```python
from build123d import *

# Parameters (mm, degrees)
GOBLET_SHELL_T                     = -4
SKETCH2_R                          = 44
CUT_TO_FIT_WITH_BLADE_CASING_DEPTH = 10


with BuildPart() as part:
    # Sketch1 → Goblet Revolve (revolve)
    with BuildSketch(Plane.XY, mode=Mode.PRIVATE) as goblet_revolve_sk:
        Polygon((0, 0), (48, 0), (48, 8), (60, 8), (60, 136), (0, 136), align=None)
    revolve(goblet_revolve_sk.sketch.rotate(Axis((0, 136, 0), (0, -1, 0)), 90), axis=Axis((0, 136, 0), (0, -1, 0)))

    # Goblet Shell
    goblet_shell_openings = [part.faces().sort_by_distance(p)[0] for p in [
        (0, 136, 0),
    ]]
    offset(amount=GOBLET_SHELL_T, openings=goblet_shell_openings, kind=Kind.INTERSECTION)

    # Sketch2 → Cut to Fit with Blade Casing (cut)
    with BuildSketch(Plane(origin=(0, 4, 0), x_dir=(1, 0, 0), z_dir=(0, 1, 0))):
        with Locations(Location((0, 0, 0), (0, 0, 270))):
            Circle(SKETCH2_R)
    extrude(amount=-CUT_TO_FIT_WITH_BLADE_CASING_DEPTH, mode=Mode.SUBTRACT)


solid = part.part
```
Geometry: final body of the model. Coordinates: model frame, mm. A direction names the side the tool comes from. Round coordinates to 2 decimals unless told otherwise and drop trailing zeros. Order: outer loops, then holes, each group sorted by start corner. A loop starts at its lowest first (then second) coordinate and runs counter-clockwise, first axis right, second up. Notation, with made-up numbers: (0.5, 80) -> (58.5, 80) arc R31 cw to (58.5, 116) -> close; hole circle Ø2 at (-39.5, -22). An arc over 180 degrees is marked (long way). Use one line per item in the form item = value. Start each with the question number.
1. Cut plane B-B (z = 0). Return the cut outline in (x, y), then the cut area to 3 significant figures.
2. Cut plane C-C (y = 50.5). Return the cut outline in (x, z), then the cut area to 3 significant figures.
3. Cut plane A-A (x = 0). Return the cut outline in (y, z).
4. Draft query along X for faces 1 (the face through (49.68, 74.87, 25.84)), 2 (the face through (-50.59, 72.9, 32.26)), 3 (the face through (-40, 8, 27)). Return one class per face: pulls with the +X half, pulls with the -X half, needs draft (parallel to the pull), parting line crosses it, or undercut.
5. Line query: probe 1 along X at (y, z) = (1.3, 0); probe 2 along Z at (x, y) = (-2, 114.5); probe 3 along X at (y, z) = (86, 0). Output: solid intervals per line, ascending.
6. Cut plane D-D (x = 52). Return the cut outline in (y, z).
7. Reachability of faces 4 (the face through (37, 12, -25)), 5 (the face through (-14.418, 4.056, 45.783)), 6 (the face through (40, 136, 40)) from +Z, -Z, +X, -X, +Y, -Y: full face, straight path, thin tool, end or side. Return the list, or none.
8. Pin query (flat end, axial travel): pin 1 Ø10 at (x, z) = (45.5, 2) entering from +Y; pin 2 Ø5 at (y, z) = (107, -11) entering from -X; pin 3 Ø8 at (x, z) = (7.5, -39) entering from -Y; pin 4 Ø8 at (x, y) = (26.5, 18.5) entering from +Z. Return the tip coordinate at first contact, or that it passes through.
Solution:
q1.outline = (-60, 8) -> (-48, 8) -> (-48, 0) -> (-44, 0) -> (-44, 12) -> (-56, 12) -> (-56, 136) -> (-60, 136) -> close; (44, 0) -> (48, 0) -> (48, 8) -> (60, 8) -> (60, 136) -> (56, 136) -> (56, 12) -> (44, 12) -> close
q1.area = 1,180 mm^2
q2.outline = circle Ø120 at (0, 0); hole circle Ø112 at (0, 0)
q2.area = 1,460 mm^2
q3.outline = (0, -48) -> (8, -48) -> (8, -60) -> (136, -60) -> (136, -56) -> (12, -56) -> (12, -44) -> (0, -44) -> close; (0, 44) -> (12, 44) -> (12, 56) -> (136, 56) -> (136, 60) -> (8, 60) -> (8, 48) -> (0, 48) -> close
q4.face_1 = undercut
q4.face_2 = parting line crosses it
q4.face_3 = needs draft
q5.probe_1 = -48 to -44, 44 to 48
q5.probe_2 = -59.97 to -55.96, 55.96 to 59.97
q5.probe_3 = -60 to -56, 56 to 60
q6.outline = (8, -29.93) -> (136, -29.93) -> (136, -20.78) -> (12, -20.78) -> (12, 20.78) -> (136, 20.78) -> (136, 29.93) -> (8, 29.93) -> close
q7.face_4 = +Y
q7.face_5 = -Y
q7.face_6 = +Z, -Z, +X, -X, +Y
q8.pin_1 = 12
q8.pin_2 = -59.39
q8.pin_3 = through
q8.pin_4 = 55.62
